Geometry check sheet. Reference: the model listing, model coordinates, mm. Give positions to 0.01 mm unless a question says otherwise; leave off trailing zeros. Order: outer loops, then holes, each group sorted by start corner. A loop starts at its lowest first (then second) coordinate and runs counter-clockwise, first axis right, second up. Notation, with made-up numbers: M -4,31 L 29,31 A14 ccw 29,38 Z; hole C 18,31.25 d3. An arc over 180 degrees is marked long. Put each result on its own line as item: value. Start each with the question number.
Q1. Section check A-A on z = 8.25. Record the cut outline in (x, y).
Q2. Go/stop test with a flat-tipped pin: pin 1 (4 mm diameter, centred on x = -49, y = 33, fed in from -Z). Record where the tip stops, or that it passes through.
Q3. Material ranges on L1, parallel to Y at x = 56, z = 5.25; L2, parallel to Y at x = 70.5, z = 8; L3, parallel to X at y = 50, z = 6.5, recorded low to high.
```python
from build123d import *

# Parameters (mm, degrees)
F0_W     = 194
F0_H     = 117
F1_DEPTH = 10
F2_R     = 5
F3_R     = 5
F4_R     = 5


with BuildPart() as f1:
    # F0 (on Top) → F1 (new body)
    with BuildSketch(Plane.XY):
        Rectangle(F0_W, F0_H)
    extrude(amount=F1_DEPTH)

    # F2
    f2_edges = [f1.edges().sort_by_distance(p)[0] for p in [
        (0, -58.5, 10),
    ]]
    fillet(f2_edges, radius=F2_R)

    # F3
    f3_edges = [f1.edges().sort_by_distance(p)[0] for p in [
        (0, -58.5, 5),
        (97, -57.035534, 8.535534),
    ]]
    fillet(f3_edges, radius=F3_R)

    # F4
    f4_edges = [f1.edges().sort_by_distance(p)[0] for p in [
        (97, 2.5, 5),
        (95.535534, 58.5, 8.535534),
        (-97, -57.035534, 8.535534),
    ]]
    fillet(f4_edges, radius=F4_R)


solid = f1.part
```
Results found:
1. outline: M -95.8,-53.5 A3.8 ccw -92,-57.3 L 92,-57.3 A3.8 ccw 95.8,-53.5 L 95.8,53.5 A3.8 ccw 92,57.3 L -95.8,57.3 Z
2. pin 1: stops at z = 0
3. L1: y = -58.49 to 58.49
3. L2: y = -57.5 to 57.5
3. L3: x = -96.77 to 96.77
